The model under review builds one solid part; all positions refer to its coordinate system, in mm. Coordinates: 2 decimals unless noted, no trailing zeros. Loops run counter-clockwise (first coordinate to the right, second up) from the corner with the lowest first, then second, coordinate; pieces in that order, holes last. Notation, with made-up numbers: M 75.5,82.5 L 94.5,82.5 A30 ccw 94.5,107.5 Z; hole C 57.25,14.5 d2. An arc over 180 degrees is marked long. Write item = value, one per line. Start each with the question number.
Q1. Wall thickness on probe 1 along X at (y, z) = (25.5, 1.3); probe 2 along X at (y, z) = (73.5, 2.55); probe 3 along X at (y, z) = (27.5, 1.35): over which ranges is each line inside the solid? List them lowest first.
Q2. We need section D-D on z = 2.35. Count the separate pieces of the cut face and the enclosed holes in it, and give its area (3 significant figures).
Q3. We need section B-B on x = -152.5. Give the boundary of the cut face in (y, z) (3 decimals), and give its area (3 significant figures).
Q4. Clearance check with a flat-ended pin moving along its axis: pin 1 Ø8.5 at (x, y) = (-212.77, 125.09) entering from -Z. State where the tip first meets the part, or that it passes through.
Q5. We need section C-C on x = -214. Give the boundary of the cut face in (y, z) (1 decimal), and give its area (3 significant figures).
Q6. We need section A-A on y = 92. Give the boundary of the cut face in (x, z) (3 decimals).
from build123d import *

# Parameters (mm, degrees)
SKETCH1_R           = 4.7625
BOSS_EXTRUDE1_DEPTH = 3.175
SKETCH2_R           = 44.45
CUT_EXTRUDE1_DEPTH  = 4.175


with BuildPart() as part:
    # Sketch1 → Boss-Extrude1 (new body)
    with BuildSketch(Plane.XY):
        with BuildLine():
            Line((-230.997719316, 150.485716341), (-103.997719316, 150.485716341))
            ThreePointArc((-103.997719316, 150.485716341), (-95.017463195, 146.765972462), (-91.297719316, 137.785716341))
            Line((-91.297719316, 137.785716341), (-91.297719316, 10.785716341))
            ThreePointArc((-91.297719316, 10.785716341), (-95.017463195, 1.80546022), (-103.997719316, -1.914283659))
            Line((-103.997719316, -1.914283659), (-230.997719316, -1.914283659))
            ThreePointArc((-230.997719316, -1.914283659), (-239.977975437, 1.80546022), (-243.697719316, 10.785716341))
            Line((-243.697719316, 10.785716341), (-243.697719316, 137.785716341))
            ThreePointArc((-243.697719316, 137.785716341), (-239.977975437, 146.765972462), (-230.997719316, 150.485716341))
        make_face()
        with Locations((-122.222219316, 125.085716341)):
            Circle(SKETCH1_R, mode=Mode.SUBTRACT)
        with Locations((-212.773219316, 125.085716341)):
            Circle(SKETCH1_R, mode=Mode.SUBTRACT)
        with Locations((-212.773219316, 23.485716341)):
            Circle(SKETCH1_R, mode=Mode.SUBTRACT)
        with Locations((-122.222219316, 23.485716341)):
            Circle(SKETCH1_R, mode=Mode.SUBTRACT)
    extrude(amount=BOSS_EXTRUDE1_DEPTH)

    # Sketch2 → Cut-Extrude1 (cut, through all)
    with BuildSketch(Plane.XY.offset(3.175)):
        with Locations((-167.497719316, 74.285716341)):
            Circle(SKETCH2_R)
    extrude(amount=-CUT_EXTRUDE1_DEPTH, mode=Mode.SUBTRACT)


solid = part.part
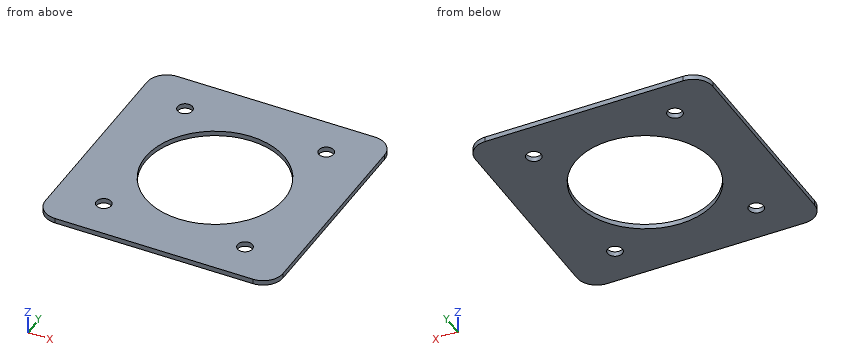
Returned:
q1.probe_1 = -243.7 to -217.09, -208.46 to -126.54, -117.91 to -91.3
q1.probe_2 = -243.7 to -211.94, -123.05 to -91.3
q1.probe_3 = -243.7 to -215.34, -210.21 to -124.78, -119.66 to -91.3
q2.separate_pieces = 1
q2.enclosed_holes = 5
q2.area = 16,600 mm^2
q3.outline = M -1.914,0 L 32.442,0 L 32.442,3.175 L -1.914,3.175 Z; M 116.129,0 L 150.486,0 L 150.486,3.175 L 116.129,3.175 Z
q3.area = 218 mm^2
q4.pin_1 = through
q5.outline = M -1.9,0 L 18.9,0 L 18.9,3.2 L -1.9,3.2 Z; M 28.1,0 L 120.5,0 L 120.5,3.2 L 28.1,3.2 Z; M 129.7,0 L 150.5,0 L 150.5,3.2 L 129.7,3.2 Z
q5.area = 425 mm^2
q6.outline = M -243.698,0 L -208.265,0 L -208.265,3.175 L -243.698,3.175 Z; M -126.73,0 L -91.298,0 L -91.298,3.175 L -126.73,3.175 Z
